```python
from build123d import *

# Parameters (mm, degrees)
SKETCH1_R            = 4
BOSS_EXTRUDE1_DEPTH  = 13
M4_CLEARANCE_HOLE1_D = 5


with BuildPart() as part:
    # Sketch1 → Boss-Extrude1 (new body)
    with BuildSketch(Plane(origin=(0, 0, 0), x_dir=(1, 0, 0), z_dir=(0, 1, 0))):
        with BuildLine():
            Line((-15, 0), (-15, -10))
            Line((-15, -10), (-27.5, -10))
            Line((-27.5, -10), (-27.5, -15))
            Line((-27.5, -15), (27.5, -15))
            Line((27.5, -15), (27.5, -10))
            Line((27.5, -10), (15, -10))
            Line((15, -10), (15, 0))
            ThreePointArc((15, 0), (0, 15), (-15, 0))
        make_face()
        with Locations(Location((0, 0, 0), (0, 0, 90))):
            Circle(SKETCH1_R, mode=Mode.SUBTRACT)
    extrude(amount=BOSS_EXTRUDE1_DEPTH)

    # M4 Clearance Hole1 (through all)
    with Locations(Plane(origin=(0, 0, 10), x_dir=(-1, 0, 0), z_dir=(0, 0, -1))):
        with Locations((-20.935, 6.5), (20.935, 6.5)):
            Hole(M4_CLEARANCE_HOLE1_D / 2)


solid = part.part
```
Source: CAD feature listing. Evaluate the final solid. Frame: model axes, mm. A direction names the side the tool comes from. Round coordinates to 2 decimals unless told otherwise and drop trailing zeros. Order: outer loops, then holes, each group sorted by start corner. A loop starts at its lowest first (then second) coordinate and runs counter-clockwise, first axis right, second up. Notation, with made-up numbers: (46, 86) -> (54, 86) arc R14 cw to (54, 99) -> close; hole circle Ø4 at (-22, -24). An arc over 180 degrees is marked (long way). Use CSV: the item, a comma, the result in double quotes.
(1) Pull-direction query (Z, two-part tool) for faces 4 (the face through (0, 6, -15)), 5 (the face through (0, 6, 15)), 6 (the face through (0, 0, 6)), 7 (the face through (3.905, 6.409, 0.867)); classes: +Z half, -Z half, draft (parallel to the pull), parting line (faces both ways), or undercut.
Report:
face 4,"-Z half"
face 5,"+Z half"
face 6,"draft"
face 7,"undercut"
(2) Section B-B on x = 0. Return the cut outline in (y, z).
Report:
outline,"(0, -15) -> (13, -15) -> (13, -4) -> (0, -4) -> close; (0, 4) -> (13, 4) -> (13, 15) -> (0, 15) -> close"
(3) Access query for faces 1 (the face through (22.279, 8.608, 12.535)), 2 (the face through (-15, 6, 5)), 3 (the face through (24, 6, 10)). Directions: +Z, -Z, +X, -X, +Y, -Y. A direction counts if a zero-diameter tool reaches every point of the face in a straight line with its end or side. Return the directions, or none.
Report:
face 1,"+Z, -Z"
face 2,"-Z, -X, +Y, -Y"
face 3,"-Z, +X, +Y, -Y"
(4) Section D-D on x = -24. Return the cut outline in (y, z), and give its area (3 significant figures).
Report:
outline,"(0, 10) -> (13, 10) -> (13, 15) -> (0, 15) -> close"
area,"65.0 mm^2"
(5) Section C-C on z = 1.75. Return the cut outline in (x, y).
Report:
outline,"(-15, 0) -> (-3.6, 0) -> (-3.6, 13) -> (-15, 13) -> close; (3.6, 0) -> (15, 0) -> (15, 13) -> (3.6, 13) -> close"
(6) First-contact query: pin 1 Ø1.5 at (x, y) = (14, 3) entering from -Z; pin 2 Ø3 at (y, z) = (4, 3) entering from -X; pin 3 Ø4.5 at (x, y) = (-20.935, 6.5) entering from -Z; pin 4 Ø2 at (y, z) = (5, -7.5) entering from -X. Flat tips, straight axial feed; report the tip coordinate or a pass-through.
Report:
pin 1,"z = -7.03"
pin 2,"x = -15"
pin 3,"through"
pin 4,"x = -13.52"
(7) Ray query, L1, parallel to X at y = 5.75, z = 13; L2, parallel to X at y = 10.5, z = 0; L3, parallel to X at y = 5.25, z = 11.75. Return the intervals inside material, ascending.
Report:
L1,"-27.5 to -23.32, -18.55 to 18.55, 23.32 to 27.5"
L2,"-15 to -4, 4 to 15"
L3,"-27.5 to -23.1, -18.77 to 18.77, 23.1 to 27.5"
(8) Section A-A on y = 6.5. Return the cut outline in (x, z) (3 decimals), and give its area (3 significant figures).
Report:
outline,"(-27.5, 10) -> (-23.435, 10) -> (-23.435, 15) -> (-27.5, 15) -> close; (-18.435, 10) -> (-15, 10) -> (-15, 0) arc R15 ccw to (15, 0) -> (15, 10) -> (18.435, 10) -> (18.435, 15) -> (-18.435, 15) -> close; (23.435, 10) -> (27.5, 10) -> (27.5, 15) -> (23.435, 15) -> close; hole circle Ø8 at (0, 0)"
area,"828 mm^2"
